Part model, mm, in its own coordinate system. A direction names the side the tool comes from. Round coordinates to 2 decimals unless told otherwise and drop trailing zeros. Loops run counter-clockwise (first coordinate to the right, second up) from the corner with the lowest first, then second, coordinate; pieces in that order, holes last. Notation, with made-up numbers: (76.25, 79.5) - (122.25, 79.5) arc R30 cw to (122.25, 109.5) - close; hole circle Ø6 at (-17.75, -7). An arc over 180 degrees is marked (long way). Put each result on its own line as item: value.
Autodesk Inventor part; units mm, degrees
ref_plane "YZ Plane" through (0, 0, 0) normal (1, 0, 0) x (0, 1, 0)
ref_plane "XZ Plane" through (0, 0, 0) normal (0, 1, 0) x (-1, 0, 0)
ref_plane "XY Plane" through (0, 0, 0) normal (0, 0, 1) x (1, 0, 0)
sketch "Sketch1" plane through (0, 0, 0) normal (0, 1, 0) x (-1, 0, 0)
  line L0 (-21.2777, 25.6513) -> (-98.2777, 25.6513)
  line L1 (-98.2777, 25.6513) -> (-98.2777, -79.3487)
  line L2 (-98.2777, -79.3487) -> (-21.2777, -79.3487)
  line L3 (-21.2777, -79.3487) -> (-21.2777, 25.6513)
  point P0 (0, 0)
  dimension "d0" = 77
  dimension "d42" = 105
extrude "Extrusion1" add sketch "Sketch1" along normal blind 1.5
sketch "Sketch5" plane through (0, 0, 0) normal (0, -1, 0) x (1, 0, 0)
  line L0 (98.2777, 25.6513) -> (98.2777, -79.3487)
  line L1 (21.2777, 25.6513) -> (98.2777, 25.6513)
  line L2 (21.2777, -79.3487) -> (21.2777, 25.6513)
  line L3 (98.2777, -79.3487) -> (21.2777, -79.3487)
  line L4 (96.7777, 24.1513) -> (96.7777, -77.8487)
  line L5 (96.7777, -77.8487) -> (22.7777, -77.8487)
  line L6 (22.7777, -77.8487) -> (22.7777, 24.1513)
  line L7 (22.7777, 24.1513) -> (96.7777, 24.1513)
  point P0 (0, 0)
  dimension "d26" = 1.5
extrude "Extrusion7" add sketch "Sketch5" along normal blind 21.26
fillet "Fillet2" radius 2 4 edges at (21.2777, -9.88, -79.3487) (98.2777, -9.88, -79.3487) (98.2777, -9.88, 25.6513) (21.2777, -9.88, 25.6513)
sketch "Sketch8" plane through (21.2777, -21.26, -77.3487) normal (-1, 0, 0) x (0, 0, 1)
  line L0 (55.5, 8.76) -> (45.5, 8.76) construction
  line L1 (55.5, 11.26) -> (45.5, 11.26)
  line L2 (45.5, 6.26) -> (55.5, 6.26)
  arc A0 (55.5, 6.26) -> (55.5, 11.26) centre (55.5, 8.76) ccw
  arc A1 (45.5, 11.26) -> (45.5, 6.26) centre (45.5, 8.76) ccw
  line L3 (101, 0) -> (0, 0)
  line L4 (101, 0) -> (0, 0) construction
  line L5 (46.5661, 0) -> (44.4339, 17.52) construction
  line L6 (0, 22.76) -> (101, 22.76)
  line L7 (0, 22.76) -> (101, 22.76) construction
  line L8 (0, 0) -> (0, 22.76) construction
  line L9 (101, 22.76) -> (101, 0)
  line L10 (0, 0) -> (0, 22.76)
  circle A2 centre (50.054, 7.7768) radius 1.7526
  point P0 (50.5, 8.76)
  point P1 (50.5, 8.76)
  dimension "d2" = 1.5
  dimension "d51" = 10
  dimension "d52" = 5
  dimension "d282" = 14
extrude "Extrusion9" cut sketch "Sketch8" against normal blind 10 contours A0 L2 A2 A1 L1 | L2 A2 picked at (50.5802, 7.7897)
sketch "Sketch9" plane through (0, 1.5, 0) normal (0, 1, 0) x (1, 0, 0)
  line L0 (35.2777, -19.1513) -> (78.2777, -19.1513)
  line L1 (81.2777, -16.1513) -> (81.2777, 50.8487)
  line L2 (78.2777, 53.8487) -> (35.2777, 53.8487)
  line L3 (32.2777, 50.8487) -> (32.2777, -16.1513)
  arc A0 (32.2777, -16.1513) -> (35.2777, -19.1513) centre (35.2777, -16.1513) ccw
  arc A1 (78.2777, -19.1513) -> (81.2777, -16.1513) centre (78.2777, -16.1513) ccw
  arc A2 (81.2777, 50.8487) -> (78.2777, 53.8487) centre (78.2777, 50.8487) ccw
  arc A3 (35.2777, 53.8487) -> (32.2777, 50.8487) centre (35.2777, 50.8487) ccw
  line L4 (98.2777, -25.6513) -> (98.2777, 79.3487)
  line L5 (21.2777, -25.6513) -> (98.2777, -25.6513)
  line L6 (22.7777, -24.1513) -> (22.7777, 77.8487)
  point P0 (0, 0)
  point P1 (81.2777, 53.8487)
  point P2 (81.2777, -19.1513)
  point P3 (32.2777, 53.8487)
  point P4 (98.2777, -23.6513)
  point P5 (98.2777, 77.3487)
  point P6 (23.2777, -25.6513)
  point P7 (96.2777, -25.6513)
  dimension "d56" = 49
  dimension "d57" = 73
  dimension "d60" = 3
  dimension "d116" = 17
  dimension "d144" = 6.5
  dimension "d283" = 9.5
extrude "Extrusion10" cut sketch "Sketch9" against normal blind 10
chamfer "Chamfer4" distance 1 angle 45 8 edges at (33.1563, 1.5, 18.2726) (32.2777, 1.5, -17.3487) (33.1563, 1.5, -52.9701) (56.7777, 1.5, -53.8487) (80.399, 1.5, -52.9701) (81.2777, 1.5, -17.3487) (80.399, 1.5, 18.2726) (56.7777, 1.5, 19.1513)
chamfer "Chamfer5" distance 2 angle 45 8 edges at (98.2777, 1.5, -26.8487) (97.6919, 1.5, -78.763) (59.7777, 1.5, -79.3487) (21.8635, 1.5, -78.763) (21.2777, 1.5, -26.8487) (21.8635, 1.5, 25.0655) (59.7777, 1.5, 25.6513) (97.6919, 1.5, 25.0655)
sketch "Sketch17" plane through (23.2777, -21.26, 25.6513) normal (0, 0, 1) x (1, 0, 0)
  line L0 (0, 20.76) -> (73, 20.76)
  line L1 (73, 0) -> (0, 0)
  line L2 (33.5, 11.26) -> (39.5, 11.26) construction
  line L3 (33.5, 9.26) -> (39.5, 9.26)
  line L4 (39.5, 13.26) -> (33.5, 13.26)
  arc A0 (33.5, 13.26) -> (33.5, 9.26) centre (33.5, 11.26) ccw
  arc A1 (39.5, 9.26) -> (39.5, 13.26) centre (39.5, 11.26) ccw
  line L5 (0, 0) -> (0, 20.76)
  line L6 (73, 20.76) -> (73, 0)
  point P0 (-23.2777, 21.26)
  point P1 (36.5, 11.26)
  dimension "d167" = 6
  dimension "d168" = 4
  dimension "d169" = 9.5
  dimension "d170" = 11.26
extrude "Extrusion17" cut sketch "Sketch17" against normal blind 4 contours A0 L4 A1 L3
chamfer "Chamfer6" distance 1 angle 45 4 edges at (59.7777, -8, 25.6513) (64.7777, -10, 25.6513) (59.7777, -12, 25.6513) (54.7777, -10, 25.6513)
sketch "Sketch18" plane through (0, 1.5, 0) normal (0, 1, 0) x (1, 0, 0)
  line L0 (96.2777, 77.3487) -> (96.2777, -23.6513)
  line L1 (82.2777, -16.1513) -> (96.2777, -16.1513)
  line L2 (81.2777, 50.8487) -> (82.2777, 50.8487)
  line L3 (96.7777, -24.1513) -> (96.7777, 77.8487)
  circle A0 centre (88.7777, 21.3487) radius 3.25
  circle A1 centre (88.7777, 40.3987) radius 3.25
  line L4 (96.2777, -23.6513) -> (23.2777, -23.6513)
  point P0 (0, 0)
  point P1 (96.7777, -22.1513)
  point P2 (96.7777, 75.8487)
  point P3 (97.2777, 77.3487)
  point P4 (97.2777, -26.6513)
  dimension "d178" = 6.5
  dimension "d179" = 6.5
  dimension "d191" = 7.5
  dimension "d192" = 7.5
  dimension "d275" = 19.05
  dimension "d276" = 45
extrude "Extrusion18" cut sketch "Sketch18" against normal blind 10
sketch "Sketch19" plane through (0, 1.5, 0) normal (0, 1, 0) x (1, 0, 0)
  circle A0 centre (88.7777, 40.3987) radius 3.25
  circle A1 centre (88.7777, 21.3487) radius 3.25
  arc A2 (31.2777, -16.1513) -> (35.2777, -20.1513) centre (35.2777, -16.1513) ccw
  line L0 (31.2777, 50.8487) -> (31.2777, -16.1513)
  arc A3 (35.2777, 54.8487) -> (31.2777, 50.8487) centre (35.2777, 50.8487) ccw
  line L1 (78.2777, 54.8487) -> (35.2777, 54.8487)
  arc A4 (82.2777, 50.8487) -> (78.2777, 54.8487) centre (78.2777, 50.8487) ccw
  line L2 (82.2777, -16.1513) -> (82.2777, 50.8487)
  arc A5 (78.2777, -20.1513) -> (82.2777, -16.1513) centre (78.2777, -16.1513) ccw
  line L3 (35.2777, -20.1513) -> (78.2777, -20.1513)
  line L4 (96.2777, -23.6513) -> (23.2777, -23.6513)
  line L5 (96.2777, 77.3487) -> (96.2777, -23.6513)
  line L6 (23.2777, 77.3487) -> (96.2777, 77.3487)
  line L7 (23.2777, -23.6513) -> (23.2777, 77.3487)
  arc A6 (35.2777, 54.8487) -> (31.2777, 50.8487) centre (35.2777, 50.8487) ccw
  arc A7 (82.2777, 50.8487) -> (78.2777, 54.8487) centre (78.2777, 50.8487) ccw
  line L8 (23.2777, 77.3487) -> (96.2777, 77.3487)
  circle A8 centre (73.7777, 67.8487) radius 3.55
  line L9 (96.2777, 77.3487) -> (96.2777, -23.6513)
  line L10 (81.2777, -16.1513) -> (81.2777, 50.8487)
  line L11 (88.7777, 40.3987) -> (88.7777, 73.4928)
  line L12 (96.7777, 75.8487) -> (96.7777, -22.1513)
  line L13 (24.7777, 77.8487) -> (94.7777, 77.8487)
  line L14 (82.2777, -16.1513) -> (82.2777, 50.8487)
  line L15 (82.2777, 43.5388) -> (96.2777, 43.5388)
  line L16 (87.0277, -12.4013) -> (91.5277, -12.4013)
  line L17 (92.5277, -11.4013) -> (92.5277, -2.9013)
  line L18 (91.5277, -1.9013) -> (87.0277, -1.9013)
  line L19 (86.0277, -2.9013) -> (86.0277, -11.4013)
  line L20 (86.0277, -12.4013) -> (92.5277, -1.9013) construction
  line L21 (92.5277, -12.4013) -> (86.0277, -1.9013) construction
  arc A9 (86.0277, -11.4013) -> (87.0277, -12.4013) centre (87.0277, -11.4013) ccw
  arc A10 (91.5277, -12.4013) -> (92.5277, -11.4013) centre (91.5277, -11.4013) ccw
  arc A11 (92.5277, -2.9013) -> (91.5277, -1.9013) centre (91.5277, -2.9013) ccw
  arc A12 (87.0277, -1.9013) -> (86.0277, -2.9013) centre (87.0277, -2.9013) ccw
  line L22 (77.1824, 62.3487) -> (70.6824, 72.8487) construction
  line L23 (35.0277, 59.5987) -> (41.5277, 70.0987) construction
  line L24 (98.2777, -23.6513) -> (98.2777, 77.3487)
  circle A13 centre (45.7777, 67.8487) radius 3.55
  line L25 (22.7777, -24.1513) -> (96.7777, -24.1513)
  point P0 (0, 0)
  point P1 (86.949, 59.6109)
  point P2 (88.2777, 58.5987)
  point P3 (89.2777, -7.1513)
  point P4 (98.2777, -25.6513)
  point P5 (98.2777, 79.3487)
  dimension "d184" = 7.1
  dimension "d200" = 10.5
  dimension "d201" = 1
  dimension "d207" = 6.5
  dimension "d209" = 5.75
  dimension "d277" = 7.1
  dimension "d278" = 28
  dimension "d284" = 9.5
  dimension "d285" = 9.5
  dimension "d286" = 22.5
  dimension "d318" = 17
extrude "Extrusion19" cut sketch "Sketch19" against normal up to surface (1.5 mm away) contours A8 | A9 L19 A12 L18 A11 L17 A10 L16 | A13
sketch "Sketch34" plane through (0, 0, 0) normal (0, -1, 0) x (1, 0, 0)
  circle A0 centre (25.4777, 21.4513) radius 1.1
  circle A1 centre (25.4777, -75.1487) radius 1.1
  circle A2 centre (94.0777, -75.1487) radius 1.1
  circle A3 centre (94.0777, 21.4513) radius 1.1
  line L0 (22.7777, 24.1513) -> (96.7777, 24.1513)
  line L1 (96.7777, 24.1513) -> (96.7777, -77.8487)
  line L2 (22.7777, -14.9487) -> (22.7777, -38.7487)
  line L3 (96.7777, -77.8487) -> (22.7777, -77.8487)
  line L4 (22.7777, 24.1513) -> (22.7777, -77.8487)
  line L5 (24.7777, -75.8487) -> (94.7777, -75.8487)
  line L6 (94.7777, -75.8487) -> (94.7777, 22.1513)
  line L7 (94.7777, 22.1513) -> (24.7777, 22.1513)
  line L8 (24.7777, 22.1513) -> (24.7777, -75.8487)
  circle A4 centre (25.4777, -75.1487) radius 2.6
  circle A5 centre (25.4777, 21.4513) radius 2.6
  circle A6 centre (94.0777, -75.1487) radius 2.6
  circle A7 centre (94.0777, 21.4513) radius 2.6
  point P0 (0, 0)
  point P1 (27.4777, 19.4513)
  point P2 (92.0777, -73.1487)
  point P3 (24.7777, -72.6447)
  point P4 (24.7777, 18.9473)
  point P5 (27.9817, 22.1513)
  point P6 (91.5737, 22.1513)
  point P7 (94.7777, 18.9473)
  point P8 (94.7777, -72.6447)
  point P9 (91.5737, -75.8487)
  point P10 (27.9817, -75.8487)
  dimension "d361" = 2.2
  dimension "d362" = 2.2
  dimension "d363" = 2.2
  dimension "d364" = 2.2
  dimension "d367" = 2
  dimension "d368" = 1.5
  dimension "d369" = 1.5
  dimension "d370" = 1.5
  dimension "d371" = 1.5
fillet "Fillet6" radius 2 4 edges at (22.7777, -10.63, -77.8487) (22.7777, -10.63, 24.1513) (96.7777, -10.63, 24.1513) (96.7777, -10.63, -77.8487)
extrude "Extrusion31" add sketch "Sketch34" along normal blind 7 contours A0 L7 A5 L8 | A0 L8 A5 L7 | A7 L6 A3 L7 | L7 A3 L6 A7 | A4 L5 A1 L8 | L8 A1 L5 A4 | A6 L5 A2 L6 | L6 A2 L5 A6 | L0 L1 L3 L4 L2
sketch "Sketch35" plane through (0, -7, 0) normal (0, -1, 0) x (1, 0, 0)
  circle A0 centre (94.0777, 21.4513) radius 1.1
  circle A1 centre (94.0777, -75.1487) radius 1.1
  circle A2 centre (25.4777, 21.4513) radius 1.1
  circle A3 centre (25.4777, -75.1487) radius 1.1
  line L0 (24.7777, -72.6447) -> (24.7777, 18.9473)
  arc A4 (24.7777, 18.9473) -> (27.9817, 22.1513) centre (25.4777, 21.4513) ccw
  line L1 (27.9817, 22.1513) -> (91.5737, 22.1513)
  arc A5 (91.5737, 22.1513) -> (94.7777, 18.9473) centre (94.0777, 21.4513) ccw
  line L2 (94.7777, 18.9473) -> (94.7777, -72.6447)
  arc A6 (94.7777, -72.6447) -> (91.5737, -75.8487) centre (94.0777, -75.1487) ccw
  line L3 (91.5737, -75.8487) -> (27.9817, -75.8487)
  arc A7 (27.9817, -75.8487) -> (24.7777, -72.6447) centre (25.4777, -75.1487) ccw
  arc A8 (22.7777, -75.8487) -> (24.7777, -77.8487) centre (24.7777, -75.8487) ccw
  line L4 (94.7777, -77.8487) -> (24.7777, -77.8487)
  arc A9 (94.7777, -77.8487) -> (96.7777, -75.8487) centre (94.7777, -75.8487) ccw
  line L5 (96.7777, 22.1513) -> (96.7777, -75.8487)
  arc A10 (96.7777, 22.1513) -> (94.7777, 24.1513) centre (94.7777, 22.1513) ccw
  line L6 (24.7777, 24.1513) -> (94.7777, 24.1513)
  arc A11 (24.7777, 24.1513) -> (22.7777, 22.1513) centre (24.7777, 22.1513) ccw
  line L7 (22.7777, -75.8487) -> (22.7777, 22.1513)
  line L8 (24.7777, 24.1513) -> (94.7777, 24.1513)
  line L9 (34.7777, 24.1513) -> (34.7777, 22.1513)
  line L10 (27.9817, 22.1513) -> (91.5737, 22.1513)
  line L11 (28.7777, 22.1513) -> (28.7777, 24.1513)
  line L12 (84.2777, 24.1513) -> (84.2777, 22.1513)
  line L13 (78.2777, 24.1513) -> (78.2777, 22.1513)
  point P0 (0, 0)
  dimension "d372" = 6
  dimension "d373" = 6
  dimension "d374" = 6
  dimension "d375" = 10.5
extrude "Extrusion32" cut sketch "Sketch35" against normal up to surface (7 mm away) contours L11 L6 L9 L1 | L13 L6 L12 L1
properties part number "Frontpanel_3DPrint"
1. Probe line 1 along X through (y, z) = (-8.75, -5); line 2 along Z through (x, y) = (56, -2.5); line 3 along X through (y, z) = (-1, -71.5). List the from-to ranges inside material, lowest first. Write a range as [from, to].
A:
line 1: x = [21.28, 22.78], [96.78, 98.28]
line 2: z = [-79.35, -75.85], [22.15, 25.65]
line 3: x = [21.28, 24.78], [94.78, 98.28]
2. Band-saw the part on C-C (z = -33). List the corners of the cut face in (x, y), plus the area to 3 significant figures.
A:
outline: (21.28, -21.26) - (22.78, -21.26) - (22.78, -14.72) - (21.28, -14.72) - close; (21.28, -10.28) - (22.78, -10.28) - (22.78, -7) - (24.78, -7) - (24.78, 0) - (32.28, 0) - (32.28, 0.5) - (31.28, 1.5) - (23.28, 1.5) - (21.28, -0.5) - close; (81.28, 0) - (94.78, 0) - (94.78, -7) - (96.78, -7) - (96.78, -21.26) - (98.28, -21.26) - (98.28, -0.5) - (96.28, 1.5) - (82.28, 1.5) - (81.28, 0.5) - close
area: 122 mm²
3. Tool access for faces 5 (the cylindrical face through (33.133, 0.254, 18.249)), 6 (the cylindrical face through (26.069, -3.451, -76.076)), 7 (the flat face through (98.278, -11, -26)), 8 (the conical face through (80.57, 0.78, 18.5)): list every direction of +Z, -Z, +X, -X, +Y, -Y with a clear straight run to the whole face (end or side of a thin tool).
A:
face 5: +Y, -Y
face 6: -Y
face 7: +Z, -Z, +X, +Y, -Y
face 8: +Y
4. Band-saw the part on B-B (x = 51.5). List the corners of the cut face in (y, z), plus the area to 3 significant figures.
A:
outline: (-21.26, -79.35) - (-0.5, -79.35) - (1.5, -77.35) - (1.5, -54.85) - (0.5, -53.85) - (0, -53.85) - (0, -75.85) - (-7, -75.85) - (-7, -77.85) - (-21.26, -77.85) - close; (-21.26, 24.15) - (-7, 24.15) - (-7, 22.15) - (0, 22.15) - (0, 19.15) - (0.5, 19.15) - (1.5, 20.15) - (1.5, 23.65) - (-0.5, 25.65) - (-21.26, 25.65) - close
area: 135 mm²
5. Two-plate mould, pull along Z, no slides. Class faces 1 (the cylindrical face through (97.68, -10.73, 25.08)), 2 (the cylindrical face through (27.343, -3.451, 19.64)), 3 (the cylindrical face through (54.78, -9.96, 24.4)), 4 (the cylindrical face through (27.289, -3.451, -73.283)): pulls with the +Z half, pulls with the -Z half, needs draft (parallel to the pull), parting line crosses it, or undercut.
A:
face 1: pulls with the +Z half
face 2: undercut
face 3: needs draft
face 4: undercut
6. Pin check, flat tips, straight feed: P1, Ø8.5, axis at x = 88.78, z = -40.4, coming from the -Y side; P2, Ø21, axis at x = 49.5, z = -20.5, coming from the -Y side; P3, Ø5, axis at y = -11, z = -22.5, coming from the -X side; P4, Ø3, axis at x = 94.08, z = 21.45, coming from the -Y side. Stop position of each tip, or through.
A:
P1: stops at y = 0
P2: passes through
P3: stops at x = 21.28
P4: stops at y = -7
7. Band-saw the part on A-A (z = -13). List the corners of the cut face in (x, y).
A:
outline: (21.28, -21.26) - (22.78, -21.26) - (22.78, -7) - (24.78, -7) - (24.78, 0) - (32.28, 0) - (32.28, 0.5) - (31.28, 1.5) - (23.28, 1.5) - (21.28, -0.5) - close; (81.28, 0) - (94.78, 0) - (94.78, -7) - (96.78, -7) - (96.78, -21.26) - (98.28, -21.26) - (98.28, -0.5) - (96.28, 1.5) - (82.28, 1.5) - (81.28, 0.5) - close
